from build123d import *

# Parameters (mm, degrees)
F1_DEPTH = 6.35
F2_R     = 1.905
F3_DEPTH = 25.4


with BuildPart() as f1:
    # F0 (on Front) → F1 (new body)
    with BuildSketch(Plane.XZ):
        with BuildLine():
            ThreePointArc((27.94, 0.508), (26.600892, 3.740892), (23.368, 5.08))
            Line((23.368, 5.08), (-23.368, 5.08))
            ThreePointArc((-23.368, 5.08), (-26.600892, 3.740892), (-27.94, 0.508))
            Line((-27.94, 0.508), (-27.94, -5.08))
            Line((-27.94, -5.08), (27.94, -5.08))
            Line((27.94, -5.08), (27.94, 0.508))
        make_face()
    extrude(amount=F1_DEPTH)

    # F2 (on face) → F3 (cut)
    with BuildSketch(Plane(origin=(0, 0, -5.08), x_dir=(1, 0, 0), z_dir=(0, 0, -1))):
        with Locations((20.8915, 3.175)):
            Circle(F2_R)
        with Locations((-20.8915, 3.175)):
            Circle(F2_R)
    extrude(amount=-F3_DEPTH, mode=Mode.SUBTRACT)


solid = f1.part
Build history of the part. All positions in model axes, mm. Round coordinates to 2 decimals unless told otherwise and drop trailing zeros. Write each loop counter-clockwise with the first axis right and the second up, starting at its lowest first coordinate (ties: lowest second). Pieces come first, ordered by that corner, then holes. Notation, with made-up numbers: (-39.75, -12) - (-20.75, -12) arc R28 cw to (-20.75, 11) - close; hole circle Ø8 at (27, -31). An arc over 180 degrees is marked (long way). One line per question, with ' | ' between items.
1. Band-saw the part on A-A, the plane y = -5.75. Write the cut outline in (x, z), and give its area (3 significant figures).
Results are:
outline: (-27.94, -5.08) - (27.94, -5.08) - (27.94, 0.51) arc R4.57 ccw to (23.37, 5.08) - (-23.37, 5.08) arc R4.57 ccw to (-27.94, 0.51) - close | area: 559 mm^2
2. Drop flat-ended pins along their axis: pin 1 Ø3 at (x, z) = (21.5, 2) entering from +Y; pin 2 Ø3 at (y, z) = (-2.5, 3.5) entering from -X. Give the stop position or say it passes through.
Results are:
pin 1: y = 0 | pin 2: x = -27.69
3. Drill centre lines: line 1 along X through (y, z) = (-3.25, -0.25); line 2 along X through (y, z) = (-4, -3.5); line 3 along Y through (x, z) = (-20.5, -1). Where is each one in solid material? Low to high. Write a range as from..to.
Results are:
line 1: -27.94..-22.8, -18.99..18.99, 22.8..27.94 | line 2: -27.94..-22.61, -19.17..19.17, 22.61..27.94 | line 3: -6.35..-5.04, -1.31..0
4. Mould opens along Y. For faces 1 (the face through (0, -3, -5.08)), 2 (the face through (-19.074, -3.747, -0.071)), 3 (the face through (0, -6.35, 0)) say: released by +Y, released by -Y, zero draft, split by the parting line, or undercut.
Results are:
face 1: zero draft | face 2: undercut | face 3: released by -Y
5. Band-saw the part on B-B, the plane z = -1.25. Give the number of separate pieces and of enclosed holes in the cut face, and give its area (3 significant figures).
Results are:
separate pieces: 1 | enclosed holes: 2 | area: 332 mm^2
